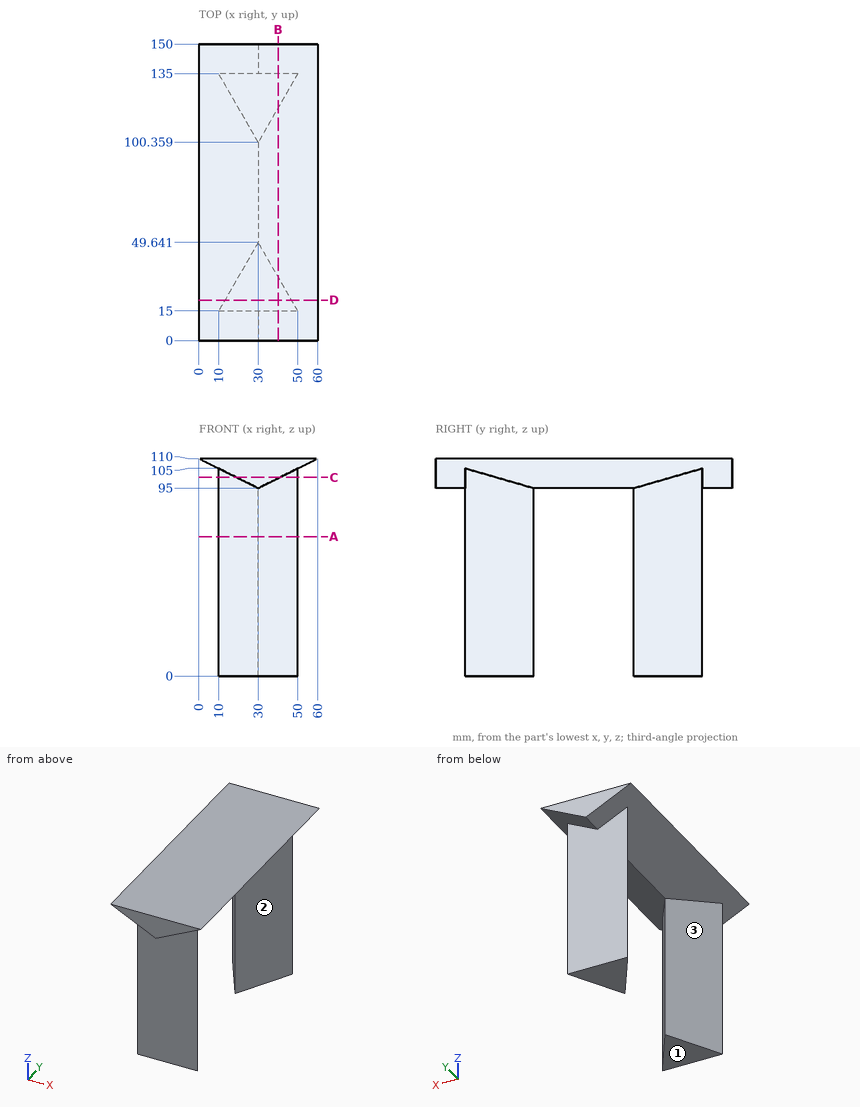
Could you check a few things on this drawing? It's one solid part, dimensions in mm from its lowest x, y, z. A direction names the side the tool comes from. Round coordinates to 2 decimals unless told otherwise and drop trailing zeros. Write each loop counter-clockwise with the first axis right and the second up, starting at its lowest first coordinate (ties: lowest second). Pieces come first, ordered by that corner, then holes.
Q1. Which directions (+Z, -Z, +X, -X, +Y, -Y) give clear straight access to the entire face, cutting with the end or side of a thin tool? Please do the marked faces 1, 2 and 3.
Q2. If we section it at C-C on z = 100.5: Write out the boundary of the cut face in (x, y).
Q3. If we section it at B-B on x = 40: Write out the boundary of the cut face in (y, z).
Q4. Please list where these lines run through material, in increasing order: probe 1 along Y at (x, z) = (39, 87.5); probe 2 along Y at (x, z) = (32.5, 20); probe 3 along Z at (x, y) = (41.5, 117).
Q5. If we section it at D-D on y = 20.5: Write out the boundary of the cut face in (x, z).
Q6. Will these pins go through, and if not, where does the flat tip stop? P1, Ø8, axis at x = 27.5, z = 54.5, coming from the -Y side; P2, Ø8, axis at x = 18.5, z = 80, coming from the +Y side; P3, Ø6, axis at y = 127, z = 71.5, coming from the +X side.
Q7. If we section it at A-A on z = 70.5: Write out the boundary of the cut face in (x, y), plus the area to 3 significant figures.
Answer below:
1. face 1: -Z, +X, -X, +Y, -Y
1. face 2: -Z, +X
1. face 3: -Z, -X
2. outline: (10, 15) - (19, 15) - (19, 0) - (41, 0) - (41, 15) - (50, 15) - (41, 30.59) - (41, 119.41) - (50, 135) - (41, 135) - (41, 150) - (19, 150) - (19, 135) - (10, 135) - (19, 119.41) - (19, 30.59) - close
3. outline: (0, 100) - (15, 100) - (15, 0) - (32.32, 0) - (32.32, 100) - (117.68, 100) - (117.68, 0) - (135, 0) - (135, 100) - (150, 100) - (150, 110) - (0, 110) - close
4. probe 1: y = 15 to 34.05, 115.95 to 135
4. probe 2: y = 15 to 45.31, 104.69 to 135
4. probe 3: z = 100.75 to 110
5. outline: (0, 110) - (13.18, 103.41) - (13.18, 0) - (46.82, 0) - (46.82, 103.41) - (60, 110) - close
6. P1: stops at y = 15
6. P2: stops at y = 135
6. P3: stops at x = 47.11
7. outline: (10, 15) - (50, 15) - (30, 49.64) - close; (10, 135) - (30, 100.36) - (50, 135) - close
7. area: 1,390 mm2
